Input: part model. Units: mm. Frame: model coordinates. Face numbers are marked on the shaded views. A direction names the side the tool comes from. Coordinates: 2 decimals unless noted, no trailing zeros. Loops run counter-clockwise (first coordinate to the right, second up) from the corner with the lowest first, then second, coordinate; pieces in that order, holes last. Notation, with made-up numbers: (40.25, 85) -> (72.25, 85) arc R26 cw to (72.25, 115) -> close; hole circle Ø4 at (58.5, 84.5). An arc over 180 degrees is marked (long way). Put each result on its own line as item: value. Start each with the question number.
1) Contact query for flat-ended pins moving along their axis: P1, Ø8, axis at x = -2, y = -62, coming from the +Z side; P2, Ø1.5, axis at x = -4.5, y = -66.5, coming from the -Z side; P3, Ø3, axis at y = -67.5, z = -6.5, coming from the -X side. Output: stop coordinate, or through.
2) Cut plane D-D (z = 9.25). Return the cut outline in (x, y).
3) Material intervals for L1, parallel to Y at x = -4.25, z = 7.5; L2, parallel to Z at x = 0.25, y = -68; L3, parallel to Z at x = -1.75, y = -61.25, sorted ascending.
4) Cut plane C-C (y = -71.25). Return the cut outline in (x, z), plus the area to 3 significant figures.
5) Cut plane A-A (y = -63.75). Return the cut outline in (x, z).
6) Set-up query: the marked faces 1 and 2. Return all of +Z, -Z, +X, -X, +Y, -Y with unobstructed straight access to the full face (end or side cutting, diameter ignored); none if empty.
7) Cut plane B-B (z = 0). Return the cut outline in (x, y).
from build123d import *

# Parameters (mm, degrees)
SKETCH1_R           = 6.38048
BOSS_EXTRUDE1_DEPTH = 8.382
BOSS_EXTRUDE2_DEPTH = 5.08
CHAMFER1_SIZE       = 2.380000066


with BuildPart() as part:
    # Sketch1 → Boss-Extrude1 (new body)
    with BuildSketch(Plane(origin=(0, -69.088, -69.088), x_dir=(1, 0, 0), z_dir=(0, 1, 0))):
        with Locations((0, -69.088)):
            Circle(SKETCH1_R)
    extrude(amount=BOSS_EXTRUDE1_DEPTH)

    # Sketch1<11> → Boss-Extrude2 (add)
    with BuildSketch(Plane(origin=(0, -69.088, -69.088), x_dir=(1, 0, 0), z_dir=(0, 1, 0))):
        Polygon((9.209764962, -74.545302509), (9.33104509, -63.840760835), (0.121280128, -58.383458325), (-9.209764962, -63.630697491), (-9.33104509, -74.335239165), (-0.121280128, -79.792541675), align=None)
    extrude(amount=-BOSS_EXTRUDE2_DEPTH)

    # Chamfer1
    chamfer1_edges = [part.edges().sort_by_distance(p)[0] for p in [
        (-6.38048, -60.706, 0),
    ]]
    chamfer(chamfer1_edges, length=CHAMFER1_SIZE)


solid = part.part
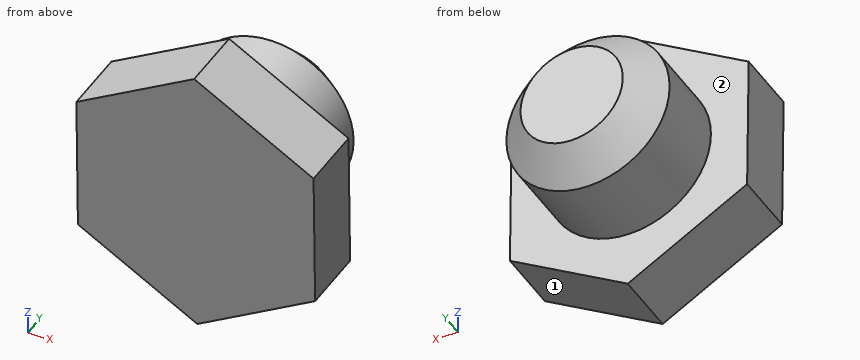
Results found:
1. P1: stops at z = 6.38
1. P2: stops at z = -5.16
1. P3: stops at x = -3.96
2. outline: (-2.58, -74.17) -> (2.47, -74.17) -> (2.47, -69.09) -> (-2.58, -69.09) -> close
3. L1: y = -74.17 to -69.09
3. L2: z = -6.38 to 6.38
3. L3: z = -4.19 to 4.19
4. outline: (-9.33, 5.25) -> (-9.21, -5.46) -> (0.12, -10.7) -> (9.33, -5.25) -> (9.21, 5.46) -> (-0.12, 10.7) -> close
4. area: 298 mm2
5. outline: circle Ø12.76 at (0, 0)
6. face 1: -Z, +X, +Y, -Y
6. face 2: +Y
7. outline: (-9.27, -74.17) -> (9.27, -74.17) -> (9.27, -69.09) -> (6.38, -69.09) -> (6.38, -63.09) -> (4, -60.71) -> (-4, -60.71) -> (-6.38, -63.09) -> (-6.38, -69.09) -> (-9.27, -69.09) -> close
